Autodesk Inventor part; units mm, degrees
ref_plane "YZ Plane" through (0, 0, 0) normal (1, 0, 0) x (0, 1, 0)
ref_plane "XZ Plane" through (0, 0, 0) normal (0, 1, 0) x (-1, 0, 0)
ref_plane "XY Plane" through (0, 0, 0) normal (0, 0, 1) x (1, 0, 0)
sketch "Эскиз3" plane through (0, 0, 0) normal (0, 0, 1) x (1, 0, 0)
  line L0 (75, -100) -> (-75, -100)
  line L1 (-75, -100) -> (-75, 100)
  line L2 (-75, 100) -> (75, 100)
  line L3 (75, 100) -> (75, -100)
  line L4 (75, -100) -> (-75, 100) construction
  line L5 (-75, -100) -> (75, 100) construction
  line L6 (-60, 85) -> (-60, -85)
  line L7 (-60, -85) -> (60, -85)
  line L8 (60, -85) -> (60, 85)
  line L9 (60, 85) -> (-60, 85)
  point P0 (0, 0)
  dimension "d11" = 150
  dimension "d12" = 200
  dimension "d13" = 15
extrude "Толщина рамки" add sketch "Эскиз3" along normal mid plane 10
sketch "Эскиз5" plane through (0, 0, 0) normal (1, 0, 0) x (0, 1, 0)
  line L0 (-100, -5) -> (100, -5)
  line L1 (0, -5) -> (-100, -31.7949)
  line L2 (-100, -31.7949) -> (-100, -5)
  line L3 (85, -5) -> (-85, -5)
  point P0 (0, 0)
  dimension "d16" = 15
  dimension "d24" = 100
extrude "Толищна подставки" add sketch "Эскиз5" along normal mid plane 20
sketch "Эскиз11" plane through (0, 0, -5) normal (0, 0, -1) x (-1, 0, 0)
  line L0 (-60, 85) -> (60, 85)
  line L1 (60, 85) -> (60, -85)
  line L2 (60, -85) -> (10, -85)
  line L3 (-10, -85) -> (-60, -85)
  line L4 (-60, -85) -> (-60, 85)
  line L5 (10, -85) -> (-10, -85)
  point P0 (0, 0)
extrude "Толщина зад. стенки" add sketch "Эскиз11" against normal blind 2
properties part number "project1"
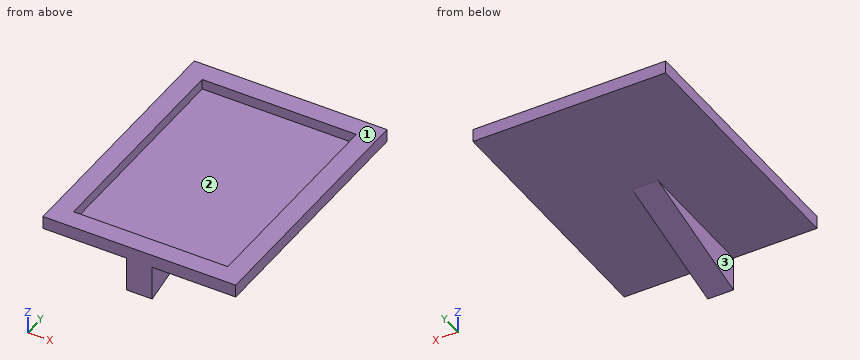
Source: CAD feature listing. Evaluate the final solid. Frame: model axes, mm. Face numbers are marked on the shaded views. Give positions to 0.01 mm unless a question says otherwise; leave off trailing zeros. Write each loop counter-clockwise with the first axis right and the second up, starting at its lowest first coordinate (ties: lowest second). Pieces come first, ordered by that corner, then holes.
1. Pull-direction query (X, two-part tool) for the marked faces 1, 2 and 3; classes: +X half, -X half, draft (parallel to the pull), parting line (faces both ways), or undercut.
2. Section query A-A (z = 1). Return the cut outline in (x, y).
3. Section query D-D (y = -10). Return the cut outline in (x, z), then the cut area to 3 significant figures.
4. Section query B-B (y = 45.5). Return the cut outline in (x, z).
5. First-contact query: pin 1 (12 mm diameter, centred on x = -35.5, y = -4.5, fed in from +Z); pin 2 (12 mm diameter, centred on x = -36.5, y = -75, fed in from -Z); pin 3 (8 mm diameter, centred on y = -55.5, z = -20, fed in from +X). Flat tips, straight axial feed; report the tip coordinate or a pass-through.
6. Material intervals for line 1 along X through (y, z) = (11, 1); line 2 along Y through (x, z) = (32, -2.5); line 3 along Z through (x, y) = (-41.5, 44.5), sorted ascending.
7. Section query C-C (x = 22). Return the cut outline in (y, z), then the cut area to 3 significant figures.
Output values:
1. face 1: draft
1. face 2: undercut
1. face 3: -X half
2. outline: (-75, -100) - (75, -100) - (75, 100) - (-75, 100) - close; hole (-60, -85) - (60, -85) - (60, 85) - (-60, 85) - close
3. outline: (-75, -5) - (-10, -5) - (-10, -7.68) - (10, -7.68) - (10, -5) - (75, -5) - (75, 5) - (60, 5) - (60, -3) - (-60, -3) - (-60, 5) - (-75, 5) - close
3. area: 594 mm2
4. outline: (-75, -5) - (75, -5) - (75, 5) - (60, 5) - (60, -3) - (-60, -3) - (-60, 5) - (-75, 5) - close
5. pin 1: stops at z = -3
5. pin 2: stops at z = -5
5. pin 3: stops at x = 10
6. line 1: x = -75 to -60, 60 to 75
6. line 2: y = -100 to -85, 85 to 100
6. line 3: z = -5 to -3
7. outline: (-100, -5) - (100, -5) - (100, 5) - (85, 5) - (85, -3) - (-85, -3) - (-85, 5) - (-100, 5) - close
7. area: 640 mm2
